Read the model definition and answer for the solid it produces. Units are mm, in the model's axes. A direction names the side the tool comes from. Coordinates: 2 decimals unless noted, no trailing zeros. Write each loop counter-clockwise with the first axis right and the second up, starting at its lowest first coordinate (ties: lowest second). Pieces come first, ordered by that corner, then holes.
Item 1: Section A-A (x = -40) is taken. Give the vertices of the cut face in (y, z).
Item 2: A tool of negligible diameter and unlimited length cuts with its end or side. For faces 1 (the face through (-1, 7.5, -12)), 2 (the face through (45.172, -0.105, -23.327)), from which of +Z, -Z, +X, -X, +Y, -Y can it reach the whole face along a straight path? Write none if from no direction.
Item 3: Determine the mould class of faces 3 (the face through (0, 0, -39.9)), 4 (the face through (31.03, -0.105, -23.534)), 5 (the face through (-1, 0, 25)), 6 (the face through (60, 0, -13)) for opening direction Z: released by +Z, released by -Z, zero draft, split by the parting line, or undercut.
Item 4: Section B-B (z = 9) is taken. State how many separate pieces and enclosed holes the cut face has, then the cut area to 3 significant figures.
Item 5: This flat-tipped pin is pushed along its axis until it touches: P1, Ø13.5, axis at x = -40, z = 3.5, coming from the -Y side. Where does it stop, or does it pass through?
Item 6: Straight lines are drawn through the part: probe 1 along Z at (x, y) = (-40, 4.5); probe 2 along Z at (x, y) = (-33, 1.75); probe 3 along X at (y, z) = (-2, -32). For each, find the intervals that lie inside material, in ascending order.
from build123d import *

# Parameters (mm, degrees)
F0_W     = 120
F0_H     = 75
F0_W_2   = 20
F0_H_2   = 20
F0_R     = 11.2835
F1_DEPTH = 7.5


with BuildPart() as f1:
    # F0 (on Front) → F1 (new body, symmetric)
    with BuildSketch(Plane.XZ):
        with Locations((0, -12.5)):
            Rectangle(F0_W, F0_H)
        with Locations((-40.000001, -29.899994)):
            Rectangle(F0_W_2, F0_H_2, mode=Mode.SUBTRACT)
        Polygon((19.999999, -39.899994), (-1e-06, -39.899994), (-20.000001, -39.899994), (-1e-06, -19.899994), align=None, mode=Mode.SUBTRACT)
        Polygon((24.057998, -30.820105), (38.199998, -16.040212), (52.341998, -30.820105), (38.199998, -45.599997), align=None, mode=Mode.SUBTRACT)
        with Locations((-39.999999, 3.504108)):
            Circle(F0_R, mode=Mode.SUBTRACT)
        with BuildLine():
            add(Edge.make_bspline(
                [(-8.488411, 18.504108), (-23.190058, 18.504108), (-15.839235, -3.995892), (-8.488411, -26.495892), (-1.137588, -3.995892), (6.213236, 18.504108), (-8.488411, 18.504108)],
                knots=[0, 0, 0, 2.094395, 2.094395, 4.18879, 4.18879, 6.283185, 6.283185, 6.283185], degree=2, weights=[1, 0.5, 1, 0.5, 1, 0.5, 1]))
        make_face(mode=Mode.SUBTRACT)
        with BuildLine():
            ThreePointArc((31.512001, -4.466328), (21.512001, -14.466328), (11.512001, -4.466328))
            Line((11.512001, -4.466328), (21.512001, 19.825672))
            Line((21.512001, 19.825672), (31.512001, -4.466328))
        make_face(mode=Mode.SUBTRACT)
    extrude(amount=F1_DEPTH, both=True)


solid = f1.part
Established:
1. outline: (-7.5, -50) - (7.5, -50) - (7.5, -39.9) - (-7.5, -39.9) - close; (-7.5, -19.9) - (7.5, -19.9) - (7.5, -7.78) - (-7.5, -7.78) - close; (-7.5, 14.79) - (7.5, 14.79) - (7.5, 25) - (-7.5, 25) - close
2. face 1: +Z, -Z, +X, -X, +Y
2. face 2: +Y, -Y
3. face 3: undercut
3. face 4: undercut
3. face 5: released by +Z
3. face 6: zero draft
4. separate pieces: 4
4. enclosed holes: 0
4. area: 1,130 mm2
5. P1: passes through
6. probe 1: z = -50 to -39.9, -19.9 to -7.78, 14.79 to 25
6. probe 2: z = -50 to -39.9, -19.9 to -5.35, 12.35 to 25
6. probe 3: x = -60 to -50, -30 to -12.1, 12.1 to 25.19, 51.21 to 60
